Verification items for the finished model (mm, model axes). Face numbers are marked on the shaded views. Give positions to 0.01 mm unless a question says otherwise; leave off trailing zeros. Write each loop counter-clockwise with the first axis right and the second up, starting at its lowest first coordinate (ties: lowest second). Pieces come first, ordered by that corner, then holes. Notation, with made-up numbers: (-3, 18.5) - (56, 18.5) arc R17 ccw to (56, 32.5) - close; hole circle Ø6 at (-27, 4). An arc over 180 degrees is marked (long way). Answer as a JSON object with one key per item and string values. Group by question number.
Item 1: Go/stop test with flat-tipped pins: pin 1 (1.2 mm diameter, centred on x = 30, z = 8, fed in from +Y); pin 2 (3 mm diameter, centred on x = 53, y = 25, fed in from -Z); pin 3 (3 mm diameter, centred on y = 15, z = 37, fed in from +X). Record where each tip stops, or that it passes through.
Item 2: Sectioned sample at C-C, the plane z = 56. Record the boundary of the cut face in (x, y), and give its area (3 significant figures).
Item 3: Draft check along X on the marked faces 1, 2, 3 and 4. Enter one of: +X half, -X half, draft (parallel to the pull), parting line (faces both ways), or undercut.
Item 4: Sectioned sample at A-A, the plane z = 21. Record the boundary of the cut face in (x, y), and give its area (3 significant figures).
Item 5: Sectioned sample at B-B, the plane y = 28.5. Record the boundary of the cut face in (x, z).
Item 6: Scan lines: line 1 along Z through (x, y) = (50, 20); line 2 along X through (y, z) = (25, 7); line 3 along Y through (x, z) = (50, 51). Record each from-to range of solid material in increasing order. Write a range as [from, to].
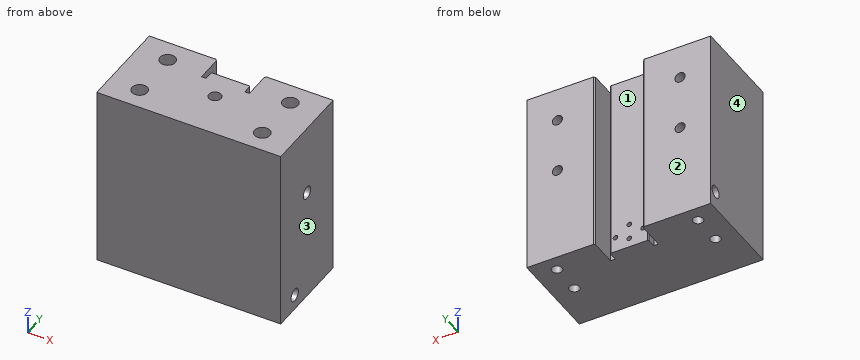
```python
from build123d import *

# Parameters (mm, degrees)
SKETCH_1_W                = 60
SKETCH_1_H                = 30
EXTRUDE_1_DEPTH           = 60
SKETCH_2_W                = 15.6
SKETCH_2_H                = 6
CUT_EXTRUDE_1_DEPTH       = 91
SKETCH_3_W                = 1.5
SKETCH_3_H                = 3
CUT_EXTRUDE_2_DEPTH       = 91
CHAMFER_1_SIZE            = 0.3
CHAMFER_2_SIZE            = 0.5
HOLE_WIZARD_M6_1_D        = 5
HOLE_WIZARD_M6_1_DEPTH    = 15
HOLE_WIZARD_M6_1_TIP      = 1.502151548
SKETCH_6_R                = 2.05
CUT_EXTRUDE_3_DEPTH       = 22.2
HOLE_WIZARD_6_0_6_1_D     = 4
HOLE_WIZARD_6_0_6_1_DEPTH = 58
HOLE_WIZARD_6_0_6_1_TIP   = 1.201721238
HOLE_WIZARD_M5_1_D        = 4.2
HOLE_WIZARD_M5_1_DEPTH    = 12.4
HOLE_WIZARD_M5_1_TIP      = 1.2618073
SKETCH_12_R               = 2
CUT_EXTRUDE_4_DEPTH       = 33
SKETCH_13_R               = 0.75
CUT_EXTRUDE_5_DEPTH       = 10
HOLE_WIZARD_M5_2_D        = 4.2
HOLE_WIZARD_M5_2_DEPTH    = 12.4
HOLE_WIZARD_M5_2_TIP      = 1.2618073
SKETCH_16_R               = 2
CUT_EXTRUDE_6_DEPTH       = 40
SKETCH_17_R               = 0.75
CUT_EXTRUDE_7_DEPTH       = 15
HOLE_WIZARD_M4_1_D        = 3.3
HOLE_WIZARD_M4_1_DEPTH    = 10.1
HOLE_WIZARD_M4_1_TIP      = 0.991420021
HOLE_WIZARD_M4_2_D        = 3.3
HOLE_WIZARD_M4_2_DEPTH    = 10.1
HOLE_WIZARD_M4_2_TIP      = 0.991420021


with BuildPart() as part:
    # 草图1 → 凸台-拉伸1 (new body)
    with BuildSketch(Plane.XY):
        with Locations((30, 15)):
            Rectangle(SKETCH_1_W, SKETCH_1_H)
    extrude(amount=EXTRUDE_1_DEPTH)

    # 草图2 → 切除-拉伸1 (cut, through all)
    with BuildSketch(Plane(origin=(0, 0, 0), x_dir=(-1, 0, 0), z_dir=(0, 0, -1))):
        with Locations((-30, 27)):
            Rectangle(SKETCH_2_W, SKETCH_2_H)
    extrude(amount=-CUT_EXTRUDE_1_DEPTH, mode=Mode.SUBTRACT)

    # 草图3 → 切除-拉伸2 (cut, through all)
    with BuildSketch(Plane(origin=(0, 0, 0), x_dir=(-1, 0, 0), z_dir=(0, 0, -1))):
        with Locations((-37.05, 22.5)):
            Rectangle(SKETCH_3_W, SKETCH_3_H)
        with Locations((-22.95, 22.5)):
            Rectangle(SKETCH_3_W, SKETCH_3_H)
    extrude(amount=-CUT_EXTRUDE_2_DEPTH, mode=Mode.SUBTRACT)

    # 倒角1
    chamfer_1_edges = [part.edges().sort_by_distance(p)[0] for p in [
        (36.3, 24, 30),
        (23.7, 24, 30),
    ]]
    chamfer(chamfer_1_edges, length=CHAMFER_1_SIZE)

    # 倒角2
    chamfer_2_edges = [part.edges().sort_by_distance(p)[0] for p in [
        (22.2, 30, 30),
        (37.8, 30, 30),
    ]]
    chamfer(chamfer_2_edges, length=CHAMFER_2_SIZE)

    # M6 螺纹孔1
    with Locations(Plane.XY.offset(60)):
        with Locations((10, 23), (50, 23), (50, 7), (10, 7)):
            Hole(HOLE_WIZARD_M6_1_D / 2, depth=HOLE_WIZARD_M6_1_DEPTH)
            with Locations((0, 0, -(HOLE_WIZARD_M6_1_DEPTH + HOLE_WIZARD_M6_1_TIP / 2))):  # 118° drill point
                Cone(0, HOLE_WIZARD_M6_1_D / 2, HOLE_WIZARD_M6_1_TIP, mode=Mode.SUBTRACT)

    # 草图6 → 切除-拉伸3 (cut)
    with BuildSketch(Plane.ZY):
        with Locations((6, 27.2)):
            Circle(SKETCH_6_R)
    extrude(amount=-CUT_EXTRUDE_3_DEPTH, mode=Mode.SUBTRACT)

    # Ø6.0 (6) 直径孔1
    with Locations(Plane.XY.offset(60)):
        with Locations((30, 15)):
            Hole(HOLE_WIZARD_6_0_6_1_D / 2, depth=HOLE_WIZARD_6_0_6_1_DEPTH)
            with Locations((0, 0, -(HOLE_WIZARD_6_0_6_1_DEPTH + HOLE_WIZARD_6_0_6_1_TIP / 2))):  # 118° drill point
                Cone(0, HOLE_WIZARD_6_0_6_1_D / 2, HOLE_WIZARD_6_0_6_1_TIP, mode=Mode.SUBTRACT)

    # M5 螺纹孔1
    with Locations(Plane(origin=(60, 0, 0), x_dir=(0, 0, -1), z_dir=(1, 0, 0))):
        with Locations((-37, 15)):
            Hole(HOLE_WIZARD_M5_1_D / 2, depth=HOLE_WIZARD_M5_1_DEPTH)
            with Locations((0, 0, -(HOLE_WIZARD_M5_1_DEPTH + HOLE_WIZARD_M5_1_TIP / 2))):  # 118° drill point
                Cone(0, HOLE_WIZARD_M5_1_D / 2, HOLE_WIZARD_M5_1_TIP, mode=Mode.SUBTRACT)

    # 草图12 → 切除-拉伸4 (cut)
    with BuildSketch(Plane(origin=(60, 0, 0), x_dir=(0, 0, -1), z_dir=(1, 0, 0))):
        with Locations((-37, 15)):
            Circle(SKETCH_12_R)
    extrude(amount=-CUT_EXTRUDE_4_DEPTH, mode=Mode.SUBTRACT)

    # 草图13 → 切除-拉伸5 (cut)
    with BuildSketch(Plane(origin=(0, 24, 0), x_dir=(1, 0, 0), z_dir=(0, 1, 0))):
        with Locations(Location((30, -3, 0), (0, 0, 180))):
            Circle(SKETCH_13_R)
        with Locations(Location((30, -8, 0), (0, 0, 180))):
            Circle(SKETCH_13_R)
    extrude(amount=-CUT_EXTRUDE_5_DEPTH, mode=Mode.SUBTRACT)

    # M5 螺纹孔2
    with Locations(Plane(origin=(60, 0, 0), x_dir=(0, 0, -1), z_dir=(1, 0, 0))):
        with Locations((-5, 8)):
            Hole(HOLE_WIZARD_M5_2_D / 2, depth=HOLE_WIZARD_M5_2_DEPTH)
            with Locations((0, 0, -(HOLE_WIZARD_M5_2_DEPTH + HOLE_WIZARD_M5_2_TIP / 2))):  # 118° drill point
                Cone(0, HOLE_WIZARD_M5_2_D / 2, HOLE_WIZARD_M5_2_TIP, mode=Mode.SUBTRACT)

    # 草图16 → 切除-拉伸6 (cut)
    with BuildSketch(Plane(origin=(60, 0, 0), x_dir=(0, 0, -1), z_dir=(1, 0, 0))):
        with Locations((-5, 8)):
            Circle(SKETCH_16_R)
    extrude(amount=-CUT_EXTRUDE_6_DEPTH, mode=Mode.SUBTRACT)

    # 草图17 → 切除-拉伸7 (cut)
    with BuildSketch(Plane(origin=(0, 24, 0), x_dir=(1, 0, 0), z_dir=(0, 1, 0))):
        with Locations(Location((25.5, -5, 0), (0, 0, 180))):
            Circle(SKETCH_17_R)
        with Locations(Location((34.5, -5, 0), (0, 0, 180))):
            Circle(SKETCH_17_R)
    extrude(amount=-CUT_EXTRUDE_7_DEPTH, mode=Mode.SUBTRACT)

    # M4 螺纹孔1
    with Locations(Plane(origin=(0, 0, 0), x_dir=(-1, 0, 0), z_dir=(0, 0, -1))):
        with Locations((-53, 25), (-53, 15), (-7, 15), (-7, 25)):
            Hole(HOLE_WIZARD_M4_1_D / 2, depth=HOLE_WIZARD_M4_1_DEPTH)
            with Locations((0, 0, -(HOLE_WIZARD_M4_1_DEPTH + HOLE_WIZARD_M4_1_TIP / 2))):  # 118° drill point
                Cone(0, HOLE_WIZARD_M4_1_D / 2, HOLE_WIZARD_M4_1_TIP, mode=Mode.SUBTRACT)

    # M4 螺纹孔2
    with Locations(Plane(origin=(0, 30, 0), x_dir=(-1, 0, 0), z_dir=(0, 1, 0))):
        with Locations((-50, 31), (-50, 49), (-10, 49), (-10, 31)):
            Hole(HOLE_WIZARD_M4_2_D / 2, depth=HOLE_WIZARD_M4_2_DEPTH)
            with Locations((0, 0, -(HOLE_WIZARD_M4_2_DEPTH + HOLE_WIZARD_M4_2_TIP / 2))):  # 118° drill point
                Cone(0, HOLE_WIZARD_M4_2_D / 2, HOLE_WIZARD_M4_2_TIP, mode=Mode.SUBTRACT)


solid = part.part
```
Geometry check:
{
 "1": {"pin 1": "y = 13.09", "pin 2": "z = 10.19", "pin 3": "x = 27"},
 "2": {"outline": "(0, 0) - (60, 0) - (60, 30) - (38.3, 30) - (37.8, 29.5) - (37.8, 21) - (36.3, 21) - (36.3, 23.7) - (36, 24) - (24, 24) - (23.7, 23.7) - (23.7, 21) - (22.2, 21) - (22.2, 29.5) - (21.7, 30) - (0, 30) - close; hole circle Ø5 at (10, 7); hole circle Ø5 at (10, 23); hole circle Ø4 at (30, 15); hole circle Ø5 at (50, 7); hole circle Ø5 at (50, 23)", "area": "1,610 mm^2"},
 "3": {"face 1": "undercut", "face 2": "draft", "face 3": "+X half", "face 4": "-X half"},
 "4": {"outline": "(0, 0) - (60, 0) - (60, 30) - (38.3, 30) - (37.8, 29.5) - (37.8, 21) - (36.3, 21) - (36.3, 23.7) - (36, 24) - (24, 24) - (23.7, 23.7) - (23.7, 21) - (22.2, 21) - (22.2, 29.5) - (21.7, 30) - (0, 30) - close; hole circle Ø4 at (30, 15)", "area": "1,680 mm^2"},
 "5": {"outline": "(0, 0) - (22.2, 0) - (22.2, 4.41) - (0, 4.41) - close; (0, 7.59) - (22.2, 7.59) - (22.2, 60) - (0, 60) - close; (37.8, 0) - (60, 0) - (60, 60) - (37.8, 60) - close; hole circle Ø3.3 at (10, 31); hole circle Ø3.3 at (10, 49); hole circle Ø3.3 at (50, 31); hole circle Ø3.3 at (50, 49)"},
 "6": {"line 1": "[0, 29.35], [32.65, 47.35], [50.65, 60]", "line 2": "[0, 5.35], [8.65, 22.2], [37.8, 51.35], [54.65, 60]", "line 3": "[0, 4.5], [9.5, 20.5], [25.5, 30]"}
}
